The listing builds one solid part. Answer for the finished solid, in the listing's coordinates (mm). Coordinates: 2 decimals unless noted, no trailing zeros. Order: outer loops, then holes, each group sorted by start corner. A loop starts at its lowest first (then second) coordinate and runs counter-clockwise, first axis right, second up. Notation, with made-up numbers: (61, -8.75) -> (92, -8.75) arc R14 cw to (92, 9.25) -> close; hole circle Ø4 at (46, 21). An arc over 180 degrees is marked (long way). One line per question, with ' | ' between items.
from build123d import *

# Parameters (mm, degrees)
SKETCH1_W           = 320
SKETCH1_H           = 40
BOSS_EXTRUDE1_DEPTH = 8
CUT_EXTRUDE1_REACH  = 10
SKETCH2_R           = 3
CUT_EXTRUDE2_REACH  = 10
SKETCH3_R           = 4
SKETCH3_R_2         = 11.5
CUT_EXTRUDE3_REACH  = 10
SKETCH4_R           = 1.75


with BuildPart() as part:
    # Sketch1 → Boss-Extrude1 (new body)
    with BuildSketch(Plane.XY):
        Rectangle(SKETCH1_W, SKETCH1_H)
    extrude(amount=BOSS_EXTRUDE1_DEPTH)

    # Sketch2 → Cut-Extrude1 (cut, up to next)
    with BuildSketch(Plane.XY.offset(8), mode=Mode.PRIVATE) as cut_extrude1_sk1:
        with Locations((-150, 10)):
            Circle(SKETCH2_R)
    cut_extrude1_tool1 = extrude(cut_extrude1_sk1.sketch, amount=-CUT_EXTRUDE1_REACH, mode=Mode.PRIVATE) & part.part
    add(cut_extrude1_tool1.solids().sort_by_distance((-150, 10, 8))[0], mode=Mode.SUBTRACT)
    # Sketch2 → Cut-Extrude1 (cut, up to next)
    with BuildSketch(Plane.XY.offset(8), mode=Mode.PRIVATE) as cut_extrude1_sk2:
        with Locations((-150, -10)):
            Circle(SKETCH2_R)
    cut_extrude1_tool2 = extrude(cut_extrude1_sk2.sketch, amount=-CUT_EXTRUDE1_REACH, mode=Mode.PRIVATE) & part.part
    add(cut_extrude1_tool2.solids().sort_by_distance((-150, -10, 8))[0], mode=Mode.SUBTRACT)
    # Sketch2 → Cut-Extrude1 (cut, up to next)
    with BuildSketch(Plane.XY.offset(8), mode=Mode.PRIVATE) as cut_extrude1_sk3:
        with Locations((150, -10)):
            Circle(SKETCH2_R)
    cut_extrude1_tool3 = extrude(cut_extrude1_sk3.sketch, amount=-CUT_EXTRUDE1_REACH, mode=Mode.PRIVATE) & part.part
    add(cut_extrude1_tool3.solids().sort_by_distance((150, -10, 8))[0], mode=Mode.SUBTRACT)
    # Sketch2 → Cut-Extrude1 (cut, up to next)
    with BuildSketch(Plane.XY.offset(8), mode=Mode.PRIVATE) as cut_extrude1_sk4:
        with Locations((150, 10)):
            Circle(SKETCH2_R)
    cut_extrude1_tool4 = extrude(cut_extrude1_sk4.sketch, amount=-CUT_EXTRUDE1_REACH, mode=Mode.PRIVATE) & part.part
    add(cut_extrude1_tool4.solids().sort_by_distance((150, 10, 8))[0], mode=Mode.SUBTRACT)

    # Sketch3 → Cut-Extrude2 (cut, up to next)
    with BuildSketch(Plane.XY.offset(8), mode=Mode.PRIVATE) as cut_extrude2_sk1:
        with Locations((-85.5, 10)):
            Circle(SKETCH3_R)
    cut_extrude2_tool1 = extrude(cut_extrude2_sk1.sketch, amount=-CUT_EXTRUDE2_REACH, mode=Mode.PRIVATE) & part.part
    add(cut_extrude2_tool1.solids().sort_by_distance((-85.5, 10, 8))[0], mode=Mode.SUBTRACT)
    # Sketch3 → Cut-Extrude2 (cut, up to next)
    with BuildSketch(Plane.XY.offset(8), mode=Mode.PRIVATE) as cut_extrude2_sk2:
        with Locations((85.5, 10)):
            Circle(SKETCH3_R)
    cut_extrude2_tool2 = extrude(cut_extrude2_sk2.sketch, amount=-CUT_EXTRUDE2_REACH, mode=Mode.PRIVATE) & part.part
    add(cut_extrude2_tool2.solids().sort_by_distance((85.5, 10, 8))[0], mode=Mode.SUBTRACT)
    # Sketch3 → Cut-Extrude2 (cut, up to next)
    with BuildSketch(Plane.XY.offset(8), mode=Mode.PRIVATE) as cut_extrude2_sk3:
        Circle(SKETCH3_R_2)
    cut_extrude2_tool3 = extrude(cut_extrude2_sk3.sketch, amount=-CUT_EXTRUDE2_REACH, mode=Mode.PRIVATE) & part.part
    add(cut_extrude2_tool3.solids().sort_by_distance((0, 0, 8))[0], mode=Mode.SUBTRACT)

    # Sketch4 → Cut-Extrude3 (cut, up to next)
    with BuildSketch(Plane.XY.offset(8), mode=Mode.PRIVATE) as cut_extrude3_sk1:
        with Locations((-15.5, 15.5)):
            Circle(SKETCH4_R)
    cut_extrude3_tool1 = extrude(cut_extrude3_sk1.sketch, amount=-CUT_EXTRUDE3_REACH, mode=Mode.PRIVATE) & part.part
    add(cut_extrude3_tool1.solids().sort_by_distance((-15.5, 15.5, 8))[0], mode=Mode.SUBTRACT)
    # Sketch4 → Cut-Extrude3 (cut, up to next)
    with BuildSketch(Plane.XY.offset(8), mode=Mode.PRIVATE) as cut_extrude3_sk2:
        with Locations((15.5, 15.5)):
            Circle(SKETCH4_R)
    cut_extrude3_tool2 = extrude(cut_extrude3_sk2.sketch, amount=-CUT_EXTRUDE3_REACH, mode=Mode.PRIVATE) & part.part
    add(cut_extrude3_tool2.solids().sort_by_distance((15.5, 15.5, 8))[0], mode=Mode.SUBTRACT)
    # Sketch4 → Cut-Extrude3 (cut, up to next)
    with BuildSketch(Plane.XY.offset(8), mode=Mode.PRIVATE) as cut_extrude3_sk3:
        with Locations((-15.5, -15.5)):
            Circle(SKETCH4_R)
    cut_extrude3_tool3 = extrude(cut_extrude3_sk3.sketch, amount=-CUT_EXTRUDE3_REACH, mode=Mode.PRIVATE) & part.part
    add(cut_extrude3_tool3.solids().sort_by_distance((-15.5, -15.5, 8))[0], mode=Mode.SUBTRACT)
    # Sketch4 → Cut-Extrude3 (cut, up to next)
    with BuildSketch(Plane.XY.offset(8), mode=Mode.PRIVATE) as cut_extrude3_sk4:
        with Locations((15.5, -15.5)):
            Circle(SKETCH4_R)
    cut_extrude3_tool4 = extrude(cut_extrude3_sk4.sketch, amount=-CUT_EXTRUDE3_REACH, mode=Mode.PRIVATE) & part.part
    add(cut_extrude3_tool4.solids().sort_by_distance((15.5, -15.5, 8))[0], mode=Mode.SUBTRACT)


solid = part.part
Item 1: Find the intervals of material crossed by L1, parallel to Y at x = 150, z = 1.5; L2, parallel to X at y = 12.5, z = 0.75; L3, parallel to X at y = 16, z = 7, in increasing order.
Computed values:
L1: y = -20 to -13, -7 to 7, 13 to 20 | L2: x = -160 to -151.66, -148.34 to -88.62, -82.38 to 82.38, 88.62 to 148.34, 151.66 to 160 | L3: x = -160 to -17.18, -13.82 to 13.82, 17.18 to 160
Item 2: Section A-A, the plane x = 150 is taken. Give the vertices of the cut face in (y, z).
Computed values:
outline: (-20, 0) -> (-13, 0) -> (-13, 8) -> (-20, 8) -> close; (-7, 0) -> (7, 0) -> (7, 8) -> (-7, 8) -> close; (13, 0) -> (20, 0) -> (20, 8) -> (13, 8) -> close
Item 3: Section B-B, the plane x = -85.5 is taken. Give the vertices of the cut face in (y, z).
Computed values:
outline: (-20, 0) -> (6, 0) -> (6, 8) -> (-20, 8) -> close; (14, 0) -> (20, 0) -> (20, 8) -> (14, 8) -> close
Item 4: Section D-D, the plane x = 0 is taken. Give the vertices of the cut face in (y, z), plus the area to 3 significant figures.
Computed values:
outline: (-20, 0) -> (-11.5, 0) -> (-11.5, 8) -> (-20, 8) -> close; (11.5, 0) -> (20, 0) -> (20, 8) -> (11.5, 8) -> close | area: 136 mm^2
Item 5: Section C-C, the plane z = 4.75 is taken. Count the separate pieces of the cut face and the enclosed holes in it, plus the area to 3 significant figures.
Computed values:
separate pieces: 1 | enclosed holes: 11 | area: 12,100 mm^2
Item 6: This flat-tipped pin is pushed along its axis until it touches: pin 1 Ø3 at (x, y) = (-15.5, -15.5) entering from +Z. Where does it stop, or does it pass through?
Computed values:
pin 1: passes through
Item 7: Determine the mould class of faces 1 (the face through (-1.5, 11.4, 4.1)), 2 (the face through (-2, -20, 4)), 3 (the face through (-160, 0, 4)) for opening direction Y: pulls with the +Y half, pulls with the -Y half, needs draft (parallel to the pull), parting line crosses it, or undercut.
Computed values:
face 1: undercut | face 2: pulls with the -Y half | face 3: needs draft
